from build123d import *

# Parameters (mm, degrees)
F0_W         = 101.6
F0_H         = 76.2
F1_DEPTH     = 127
F2_T         = -6.35
F3_T1_DEPTH  = 152.4
F3_T3_DEPTH  = 134.62
F3_T5_DEPTH  = 101.6
F3_T7_DEPTH  = 66.04
F3_T9_DEPTH  = 109.22
F3_T11_DEPTH = 88.9
F3_T13_DEPTH = 63.5
F3_S17_W     = 5.1816
F3_S17_H     = 5.1816
F3_T18_DEPTH = 5.1816
F3_S23_W     = 5.1816
F3_S23_H     = 5.1816
F3_T24_DEPTH = 5.1816
F3_T31_DEPTH = 101.6
F3_T36_DEPTH = 76.2
F3_T44_DEPTH = 76.2
F3_T49_DEPTH = 101.6
F3_T57_DEPTH = 101.6
F3_T62_DEPTH = 76.2
F3_T70_DEPTH = 101.6
F3_T75_DEPTH = 76.2


# Not quite as in the source:
# - a fillet or chamfer that OpenCascade refuses, or shapes differently, is made with other operations: its cross-section is extruded or revolved along the edge and cut away or added


with BuildPart() as f1:
    # F0 (on Top) → F1 (new body)
    with BuildSketch(Plane.XY):
        with Locations((74.7453766656, -13.2239237391)):
            Rectangle(F0_W, F0_H)
    extrude(amount=F1_DEPTH)

    # F2
    f2_openings = [f1.faces().sort_by_distance(p)[0] for p in [
        (74.745377, -13.223924, 127),
    ]]
    offset(amount=F2_T, openings=f2_openings)

    # F3: fillet of radius 5.08 on 12 edges, made by hand

    # F3_s2 → F3_t1 (cut)
    with BuildSketch(Plane.XY.offset(-12.7)):
        with BuildLine():
            ThreePointArc((29.0253766656, 24.8760762609), (25.4332742171, 23.3881787093), (23.9453766656, 19.7960762609))
            Line((23.9453766656, 19.7960762609), (23.9453766656, 24.8760762609))
            Line((23.9453766656, 24.8760762609), (29.0253766656, 24.8760762609))
        make_face()
        with BuildLine():
            ThreePointArc((29.0253766656, -51.3239237391), (25.4332742171, -49.8360261876), (23.9453766656, -46.2439237391))
            Line((23.9453766656, -46.2439237391), (23.9453766656, -51.3239237391))
            Line((23.9453766656, -51.3239237391), (29.0253766656, -51.3239237391))
        make_face()
    extrude(amount=F3_T1_DEPTH, mode=Mode.SUBTRACT)

    # F3_s4 → F3_t3 (cut)
    with BuildSketch(Plane.XY.offset(-12.7)):
        with BuildLine():
            ThreePointArc((125.5453766656, 19.7960762609), (124.057479114, 23.3881787093), (120.4653766656, 24.8760762609))
            Line((120.4653766656, 24.8760762609), (125.5453766656, 24.8760762609))
            Line((125.5453766656, 24.8760762609), (125.5453766656, 19.7960762609))
        make_face()
        with BuildLine():
            ThreePointArc((120.4653766656, -51.3239237391), (124.057479114, -49.8360261876), (125.5453766656, -46.2439237391))
            Line((125.5453766656, -46.2439237391), (125.5453766656, -51.3239237391))
            Line((125.5453766656, -51.3239237391), (120.4653766656, -51.3239237391))
        make_face()
    extrude(amount=F3_T3_DEPTH, mode=Mode.SUBTRACT)

    # F3_s6 → F3_t5 (cut)
    with BuildSketch(Plane.XZ.offset(-37.5760762609)):
        with BuildLine():
            ThreePointArc((125.5453766656, 5.08), (124.057479114, 1.4878975516), (120.4653766656, 0))
            Line((120.4653766656, 0), (125.5453766656, 0))
            Line((125.5453766656, 0), (125.5453766656, 5.08))
        make_face()
    extrude(amount=F3_T5_DEPTH, mode=Mode.SUBTRACT)

    # F3_s8 → F3_t7 (cut)
    with BuildSketch(Plane.XZ.offset(-19.7960762609)):
        with BuildLine():
            ThreePointArc((125.5453766656, 121.92), (124.057479114, 125.5121024484), (120.4653766656, 127))
            Line((120.4653766656, 127), (125.5453766656, 127))
            Line((125.5453766656, 127), (125.5453766656, 121.92))
        make_face()
    extrude(amount=F3_T7_DEPTH, mode=Mode.SUBTRACT)

    # F3_s10 → F3_t9 (cut)
    with BuildSketch(Plane.YZ.offset(11.2453766656)):
        with BuildLine():
            ThreePointArc((-51.3239237391, 121.92), (-49.8360261876, 125.5121024484), (-46.2439237391, 127))
            Line((-46.2439237391, 127), (-51.3239237391, 127))
            Line((-51.3239237391, 127), (-51.3239237391, 121.92))
        make_face()
        with BuildLine():
            ThreePointArc((24.8760762609, 121.92), (23.3881787093, 125.5121024484), (19.7960762609, 127))
            Line((19.7960762609, 127), (24.8760762609, 127))
            Line((24.8760762609, 127), (24.8760762609, 121.92))
        make_face()
    extrude(amount=F3_T9_DEPTH, mode=Mode.SUBTRACT)

    # F3_s12 → F3_t11 (cut)
    with BuildSketch(Plane.YZ.offset(30.2953766656)):
        with BuildLine():
            ThreePointArc((23.6060762609, 127), (20.0139738124, 125.5121024484), (18.5260762609, 121.92))
            Line((18.5260762609, 121.92), (18.5260762609, 127))
            Line((18.5260762609, 127), (23.6060762609, 127))
        make_face()
        with BuildLine():
            ThreePointArc((-50.0539237391, 127), (-46.4618212907, 125.5121024484), (-44.9739237391, 121.92))
            Line((-44.9739237391, 121.92), (-44.9739237391, 127))
            Line((-44.9739237391, 127), (-50.0539237391, 127))
        make_face()
    extrude(amount=F3_T11_DEPTH, mode=Mode.SUBTRACT)

    # F3_s14 → F3_t13 (cut)
    with BuildSketch(Plane.XZ.offset(-18.5260762609)):
        with BuildLine():
            ThreePointArc((25.2153766656, 127), (28.807479114, 125.5121024484), (30.2953766656, 121.92))
            Line((30.2953766656, 121.92), (30.2953766656, 127))
            Line((30.2953766656, 127), (25.2153766656, 127))
        make_face()
        with BuildLine():
            ThreePointArc((124.2753766656, 127), (120.6832742171, 125.5121024484), (119.1953766656, 121.92))
            Line((119.1953766656, 121.92), (119.1953766656, 127))
            Line((119.1953766656, 127), (124.2753766656, 127))
        make_face()
    extrude(amount=F3_T13_DEPTH, mode=Mode.SUBTRACT)


with BuildPart() as f3_tool16:
    # F3_s17 → F3_t18 (new body)
    with BuildSketch(Plane.YZ.offset(120.4653766656)):
        with Locations((22.3868762609, 124.5108)):
            Rectangle(F3_S17_W, F3_S17_H)
    extrude(amount=F3_T18_DEPTH)

    # F3_s19 → F3_t20 (revolve, cut)
    with BuildSketch(Plane(origin=(120.4653766656, 19.7960762609, 121.92), x_dir=(0, -0.7071067812, -0.7071067812), z_dir=(0, -0.7071067812, 0.7071067812))):
        with BuildLine():
            ThreePointArc((0, -5.08), (5.08, 0), (0, 5.08))
            Line((0, 5.08), (0, -5.08))
        make_face()
    revolve(axis=Axis((120.4653766656, 19.7960762609, 121.92), (1, 0, 0)), mode=Mode.SUBTRACT)


with BuildPart() as f1_1:
    add(f1.part)

    # F3_t15: cut F3_tool16
    add(f3_tool16.part, mode=Mode.SUBTRACT)


with BuildPart() as f3_tool22:
    # F3_s23 → F3_t24 (new body)
    with BuildSketch(Plane.XZ.offset(46.2439237391)):
        with Locations((123.0561766656, 124.5108)):
            Rectangle(F3_S23_W, F3_S23_H)
    extrude(amount=F3_T24_DEPTH)

    # F3_s25 → F3_t26 (revolve, cut)
    with BuildSketch(Plane(origin=(120.4653766656, -46.2439237391, 121.92), x_dir=(-0.7071067812, 0, -0.7071067812), z_dir=(-0.7071067812, 0, 0.7071067812))):
        with BuildLine():
            ThreePointArc((0, -5.08), (5.08, 0), (0, 5.08))
            Line((0, 5.08), (0, -5.08))
        make_face()
    revolve(axis=Axis((120.4653766656, -46.2439237391, 121.92), (0, -1, 0)), mode=Mode.SUBTRACT)


with BuildPart() as f1_2:
    add(f1_1.part)

    # F3_t21: cut F3_tool22
    add(f3_tool22.part, mode=Mode.SUBTRACT)


with BuildPart() as f3_tool29:
    # F3_s30 → F3_t31 (new body)
    with BuildSketch(Plane.YZ.offset(131.8953766656)):
        with BuildLine():
            ThreePointArc((23.6060762609, 127), (20.0139738124, 125.5121024484), (18.5260762609, 121.92))
            Line((18.5260762609, 121.92), (18.5260762609, 127))
            Line((18.5260762609, 127), (23.6060762609, 127))
        make_face()
    extrude(amount=-F3_T31_DEPTH)

    split(bisect_by=Plane.YZ.offset(125.5453766656), keep=Keep.BOTTOM)

    split(bisect_by=Plane.YZ.offset(119.1953766656), keep=Keep.TOP)


with BuildPart() as f3_tool34:
    # F3_s35 → F3_t36 (new body)
    with BuildSketch(Plane.XZ.offset(44.9739237391)):
        with BuildLine():
            ThreePointArc((124.2753766656, 127), (120.6832742171, 125.5121024484), (119.1953766656, 121.92))
            Line((119.1953766656, 121.92), (119.1953766656, 127))
            Line((119.1953766656, 127), (124.2753766656, 127))
        make_face()
    extrude(amount=-F3_T36_DEPTH)

    split(bisect_by=Plane.XZ.offset(-24.8760762609), keep=Keep.TOP)

    split(bisect_by=Plane.XZ.offset(-18.5260762609), keep=Keep.BOTTOM)


with BuildPart() as f3_tool29_1:
    add(f3_tool29.part)

    # F3_t39: intersect F3_tool34
    add(f3_tool34.part, mode=Mode.INTERSECT)


with BuildPart() as f1_3:
    add(f1_2.part)

    # F3_t27: cut F3_tool29
    add(f3_tool29_1.part, mode=Mode.SUBTRACT)


with BuildPart() as f3_tool42:
    # F3_s43 → F3_t44 (new body)
    with BuildSketch(Plane.XZ.offset(-31.2260762609)):
        with BuildLine():
            ThreePointArc((25.2153766656, 127), (28.807479114, 125.5121024484), (30.2953766656, 121.92))
            Line((30.2953766656, 121.92), (30.2953766656, 127))
            Line((30.2953766656, 127), (25.2153766656, 127))
        make_face()
    extrude(amount=F3_T44_DEPTH)

    split(bisect_by=Plane.XZ.offset(-24.8760762609), keep=Keep.TOP)

    split(bisect_by=Plane.XZ.offset(-18.5260762609), keep=Keep.BOTTOM)


with BuildPart() as f3_tool47:
    # F3_s48 → F3_t49 (new body)
    with BuildSketch(Plane.YZ.offset(119.1953766656)):
        with BuildLine():
            ThreePointArc((23.6060762609, 127), (20.0139738124, 125.5121024484), (18.5260762609, 121.92))
            Line((18.5260762609, 121.92), (18.5260762609, 127))
            Line((18.5260762609, 127), (23.6060762609, 127))
        make_face()
    extrude(amount=-F3_T49_DEPTH)

    split(bisect_by=Plane.YZ.offset(23.9453766656), keep=Keep.TOP)

    split(bisect_by=Plane.YZ.offset(30.2953766656), keep=Keep.BOTTOM)


with BuildPart() as f3_tool42_1:
    add(f3_tool42.part)

    # F3_t52: intersect F3_tool47
    add(f3_tool47.part, mode=Mode.INTERSECT)


with BuildPart() as f1_4:
    add(f1_3.part)

    # F3_t40: cut F3_tool42
    add(f3_tool42_1.part, mode=Mode.SUBTRACT)


with BuildPart() as f3_tool55:
    # F3_s56 → F3_t57 (new body)
    with BuildSketch(Plane.YZ.offset(17.5953766656)):
        with BuildLine():
            ThreePointArc((-50.0539237391, 127), (-46.4618212907, 125.5121024484), (-44.9739237391, 121.92))
            Line((-44.9739237391, 121.92), (-44.9739237391, 127))
            Line((-44.9739237391, 127), (-50.0539237391, 127))
        make_face()
    extrude(amount=F3_T57_DEPTH)

    split(bisect_by=Plane.YZ.offset(23.9453766656), keep=Keep.TOP)

    split(bisect_by=Plane.YZ.offset(30.2953766656), keep=Keep.BOTTOM)


with BuildPart() as f3_tool60:
    # F3_s61 → F3_t62 (new body)
    with BuildSketch(Plane.XZ.offset(-18.5260762609)):
        with BuildLine():
            ThreePointArc((25.2153766656, 127), (28.807479114, 125.5121024484), (30.2953766656, 121.92))
            Line((30.2953766656, 121.92), (30.2953766656, 127))
            Line((30.2953766656, 127), (25.2153766656, 127))
        make_face()
    extrude(amount=F3_T62_DEPTH)

    split(bisect_by=Plane.XZ.offset(51.3239237391), keep=Keep.BOTTOM)

    split(bisect_by=Plane.XZ.offset(44.9739237391), keep=Keep.TOP)


with BuildPart() as f3_tool55_1:
    add(f3_tool55.part)

    # F3_t65: intersect F3_tool60
    add(f3_tool60.part, mode=Mode.INTERSECT)


with BuildPart() as f1_5:
    add(f1_4.part)

    # F3_t53: cut F3_tool55
    add(f3_tool55_1.part, mode=Mode.SUBTRACT)


with BuildPart() as f3_tool68:
    # F3_s69 → F3_t70 (new body)
    with BuildSketch(Plane.YZ.offset(30.2953766656)):
        with BuildLine():
            ThreePointArc((-50.0539237391, 127), (-46.4618212907, 125.5121024484), (-44.9739237391, 121.92))
            Line((-44.9739237391, 121.92), (-44.9739237391, 127))
            Line((-44.9739237391, 127), (-50.0539237391, 127))
        make_face()
    extrude(amount=F3_T70_DEPTH)

    split(bisect_by=Plane.YZ.offset(125.5453766656), keep=Keep.BOTTOM)

    split(bisect_by=Plane.YZ.offset(119.1953766656), keep=Keep.TOP)


with BuildPart() as f3_tool73:
    # F3_s74 → F3_t75 (new body)
    with BuildSketch(Plane.XZ.offset(57.6739237391)):
        with BuildLine():
            ThreePointArc((124.2753766656, 127), (120.6832742171, 125.5121024484), (119.1953766656, 121.92))
            Line((119.1953766656, 121.92), (119.1953766656, 127))
            Line((119.1953766656, 127), (124.2753766656, 127))
        make_face()
    extrude(amount=-F3_T75_DEPTH)

    split(bisect_by=Plane.XZ.offset(51.3239237391), keep=Keep.BOTTOM)

    split(bisect_by=Plane.XZ.offset(44.9739237391), keep=Keep.TOP)


with BuildPart() as f3_tool68_1:
    add(f3_tool68.part)

    # F3_t78: intersect F3_tool73
    add(f3_tool73.part, mode=Mode.INTERSECT)


with BuildPart() as f1_6:
    add(f1_5.part)

    # F3_t66: cut F3_tool68
    add(f3_tool68_1.part, mode=Mode.SUBTRACT)


solid = f1_6.part
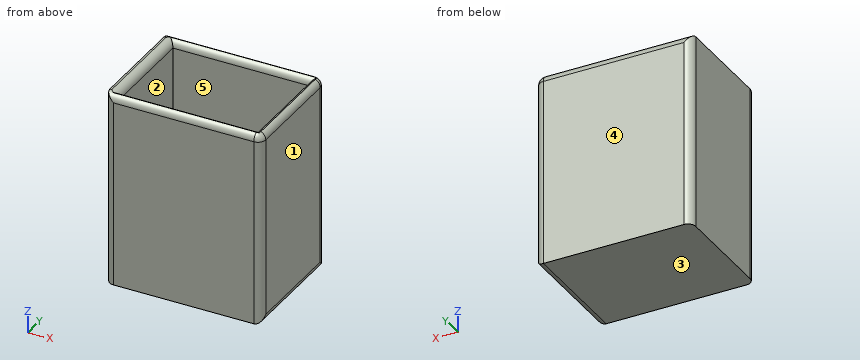
Geometry check sheet. Reference: the model listing, model coordinates, mm. Face numbers are marked on the shaded views. A direction names the side the tool comes from. Round coordinates to 2 decimals unless told otherwise and drop trailing zeros. Loops run counter-clockwise (first coordinate to the right, second up) from the corner with the lowest first, then second, coordinate; pieces in that order, holes last.
Item 1: Thickness scan on line 1 (X direction, y = -22.5, z = 58); line 2 (Y direction, x = 103, z = 40); line 3 (Z direction, x = 45, y = 11). Record the ranges inside material, lowest first.
Item 2: Cross-section at C-C on x = 67. Record the boundary of the cut face in (y, z).
Item 3: Cross-section at A-A on z = 11. Record the boundary of the cut face in (x, y).
Item 4: Gauge pin test, flat ends, axial feed: pin 1 (12 mm diameter, centred on x = 89, y = -16.5, fed in from +Z); pin 2 (3 mm diameter, centred on x = 39, y = -1.5, fed in from -Z). Record the tip position at first contact, or that the pin passes through.
Item 5: Mould release check, pull along X, two halves, no side actions. Record for the marked faces 1, 2 and 3: pulls with the +X half, pulls with the -X half, needs draft (parallel to the pull), parting line crosses it, or undercut.
Item 6: Access from +Z, -Z, +X, -X, +Y, -Y to the whole of each face (thin tool, end or side, straight path). Record for the marked faces 4 and 5.
Item 7: Cross-section at B-B on y = -41. Record the boundary of the cut face in (x, z), then the cut area to 3 significant figures.
Answer sheet:
1. line 1: x = 23.95 to 30.3, 119.2 to 125.55
1. line 2: y = -51.32 to -44.97, 18.53 to 24.88
1. line 3: z = 0 to 6.35
2. outline: (-51.32, 0) - (24.88, 0) - (24.88, 121.92) arc R5.08 ccw to (21.7, 126.63) arc R5.08 ccw to (18.53, 121.92) - (18.53, 6.35) - (-44.97, 6.35) - (-44.97, 121.92) arc R5.08 ccw to (-48.15, 126.63) arc R5.08 ccw to (-51.32, 121.92) - close
3. outline: (23.95, -46.24) arc R5.08 ccw to (29.03, -51.32) - (120.47, -51.32) arc R5.08 ccw to (125.55, -46.24) - (125.55, 19.8) arc R5.08 ccw to (120.47, 24.88) - (29.03, 24.88) arc R5.08 ccw to (23.95, 19.8) - close; hole (30.3, -44.97) - (119.2, -44.97) - (119.2, 18.53) - (30.3, 18.53) - close
4. pin 1: stops at z = 6.35
4. pin 2: stops at z = 0
5. face 1: pulls with the +X half
5. face 2: undercut
5. face 3: needs draft
6. face 4: +Z, -Z, +X, -X, +Y
6. face 5: +Z
7. outline: (23.95, 0) - (120.47, 0) arc R5.08 ccw to (125.55, 5.08) - (125.55, 121.92) arc R5.08 ccw to (122.37, 126.63) arc R5.08 ccw to (119.2, 121.92) - (119.2, 6.35) - (30.3, 6.35) - (30.3, 121.92) arc R5.08 ccw to (25.22, 127) - (23.95, 127) - close
7. area: 2,160 mm2
